from build123d import *

# Parameters (mm, degrees)
BOSS_EXTRUDE1_DEPTH     = 15.24
CUT_EXTRUDE2_DEPTH      = 2.54
CUT_EXTRUDE3_DEPTH      = 26.416
CUT_EXTRUDE4_DEPTH      = 2.54
CUT_EXTRUDE5_DEPTH      = 37.592
CUT_EXTRUDE5_DEPTH_BACK = 16.256
SKETCH6_W               = 28.095448716
SKETCH6_H               = 6.506871402
CUT_EXTRUDE6_DEPTH      = 33.782
CUT_EXTRUDE6_DEPTH_BACK = 30.988
CUT_EXTRUDE7_DEPTH      = 30.988
BOSS_EXTRUDE2_DEPTH     = 2.54


with BuildPart() as part:
    # Sketch1 → Boss-Extrude1 (new body)
    with BuildSketch(Plane(origin=(0, 0, 0), x_dir=(1, 0, 0), z_dir=(0, 1, 0))):
        Polygon((0, 0), (19.056811247, 0), (19.056811247, 6.097892911), (26.173997358, 6.097892911), (15.563225472, -28.095448716), (7.752418672, -26.383450539), (6.430712527, -32.413592092), (-14.191226065, -27.893608153), (-12.86951992, -21.8634666), (-25.576280295, -19.078357307), (-6.082744599, 6.097892911), (0, 6.097892911), align=None)
    extrude(amount=BOSS_EXTRUDE1_DEPTH)

    # Sketch2 → Cut-Extrude2 (cut)
    with BuildSketch(Plane(origin=(0, 15.24, 0), x_dir=(1, 0, 0), z_dir=(0, 1, 0))):
        Polygon((-12.86951992, -21.8634666), (7.752418672, -26.383450539), (6.430712527, -32.413592092), (-14.191226065, -27.893608153), align=None)
    extrude(amount=-CUT_EXTRUDE2_DEPTH, mode=Mode.SUBTRACT)

    # Sketch3 → Cut-Extrude3 (cut)
    with BuildSketch(Plane(origin=(12.914786435, 0, 2.830705125), x_dir=(0.214100757, 0, -0.976811582), z_dir=(0.976811582, 0, 0.214100757))):
        with BuildLine():
            Line((-29.362167954, 11.792818882), (-30.285151737, 12.7))
            Line((-30.285151737, 12.7), (-30.285151737, 6.632404251))
            Line((-30.285151737, 6.632404251), (-27.19850654, 6.632404251))
            ThreePointArc((-27.19850654, 6.632404251), (-29.99633203, 8.493128354), (-29.362167954, 11.792818882))
        make_face()
        with BuildLine():
            Line((-27.19850654, 12.7), (-30.285151737, 12.7))
            Line((-30.285151737, 12.7), (-29.362167954, 11.792818882))
            ThreePointArc((-29.362167954, 11.792818882), (-28.371580312, 12.464027615), (-27.19850654, 12.7))
        make_face()
        with BuildLine():
            ThreePointArc((-25.999973236, 9.666202125), (-26.744632367, 10.775472298), (-28.053283414, 10.506344124))
            Line((-28.053283414, 10.506344124), (-26.343729666, 8.826060127))
            ThreePointArc((-26.343729666, 8.826060127), (-26.089236367, 9.212327952), (-25.999973236, 9.666202125))
        make_face()
        with BuildLine():
            Line((-26.343729666, 8.826060127), (-28.053283414, 10.506344124))
            ThreePointArc((-28.053283414, 10.506344124), (-28.038648539, 8.811425251), (-26.343729666, 8.826060127))
        make_face()
        Polygon((-27.19850654, 6.632404251), (-30.285151737, 6.632404251), (-30.285151737, 0), (-24.111861344, 0), (-24.111861344, 6.632404251), align=None)
    extrude(amount=-CUT_EXTRUDE3_DEPTH, mode=Mode.SUBTRACT)

    # Sketch4 → Cut-Extrude4 (cut)
    with BuildSketch(Plane(origin=(0, 15.24, 0), x_dir=(1, 0, 0), z_dir=(0, 1, 0))):
        Polygon((0, 0), (0, 6.097892911), (-6.082744599, 6.097892911), (-10.804237756, 0), align=None)
        Polygon((19.056811247, 0), (24.281718113, 0), (26.173997358, 6.097892911), (19.056811247, 6.097892911), align=None)
    extrude(amount=-CUT_EXTRUDE4_DEPTH, mode=Mode.SUBTRACT)

    # Sketch5 → Cut-Extrude5 (cut, two sides)
    with BuildSketch(Plane.ZY.offset(-19.056811247)) as cut_extrude5_sk:
        with BuildLine():
            ThreePointArc((-1.900262012, 9.603435701), (-2.605255865, 10.662970793), (-3.854871247, 10.421947266))
            Line((-3.854871247, 10.421947266), (-2.243021664, 8.784924136))
            ThreePointArc((-2.243021664, 8.784924136), (-1.989411364, 9.15974511), (-1.900262012, 9.603435701))
        make_face()
        with BuildLine():
            Line((-2.243021664, 8.784924136), (-3.854871247, 10.421947266))
            ThreePointArc((-3.854871247, 10.421947266), (-3.867458021, 8.79751091), (-2.243021664, 8.784924136))
        make_face()
        with BuildLine():
            ThreePointArc((-3.048946456, 6.506871402), (-5.038116892, 7.230270846), (-6.097892911, 9.062477322))
            Line((-6.097892911, 9.062477322), (-6.097892911, 6.506871402))
            Line((-6.097892911, 6.506871402), (-3.048946456, 6.506871402))
        make_face()
        Polygon((-3.048946456, 6.506871402), (-6.097892911, 6.506871402), (-6.097892911, 0), (0, 0), (0, 6.506871402), align=None)
        with BuildLine():
            Line((-5.221516955, 11.809936977), (-6.097892911, 12.7))
            Line((-6.097892911, 12.7), (-6.097892911, 10.14439408))
            ThreePointArc((-6.097892911, 10.14439408), (-5.789305577, 11.045358842), (-5.221516955, 11.809936977))
        make_face()
        with BuildLine():
            Line((-3.048946456, 12.7), (-6.097892911, 12.7))
            Line((-6.097892911, 12.7), (-5.221516955, 11.809936977))
            ThreePointArc((-5.221516955, 11.809936977), (-4.22285816, 12.468857444), (-3.048946456, 12.7))
        make_face()
    extrude(amount=CUT_EXTRUDE5_DEPTH, mode=Mode.SUBTRACT)
    extrude(cut_extrude5_sk.sketch, amount=-CUT_EXTRUDE5_DEPTH_BACK, mode=Mode.SUBTRACT)

    # Sketch6 → Cut-Extrude6 (cut, two sides)
    with BuildSketch(Plane(origin=(0, 0, 0), x_dir=(0, 0, -1), z_dir=(1, 0, 0))) as cut_extrude6_sk:
        with Locations((-14.047724358, 3.253435701)):
            Rectangle(SKETCH6_W, SKETCH6_H)
    extrude(amount=CUT_EXTRUDE6_DEPTH, mode=Mode.SUBTRACT)
    extrude(cut_extrude6_sk.sketch, amount=-CUT_EXTRUDE6_DEPTH_BACK, mode=Mode.SUBTRACT)

    # Sketch7 → Cut-Extrude7 (cut)
    with BuildSketch(Plane(origin=(0, 15.24, 0), x_dir=(1, 0, 0), z_dir=(0, 1, 0))):
        Polygon((14.008950707, -3.834200977), (7.607295542, -3.834200977), (0.172703368, -18.672351511), (6.066325192, -20.069477121), align=None)
        Polygon((0.172703368, -18.672351511), (7.607295542, -3.834200977), (1.320524054, -3.834200977), (-6.028876319, -17.202222267), align=None)
    extrude(amount=-CUT_EXTRUDE7_DEPTH, mode=Mode.SUBTRACT)

    # Sketch8 → Boss-Extrude2 (add)
    with BuildSketch(Plane(origin=(0, 15.24, 0), x_dir=(1, 0, 0), z_dir=(0, 1, 0))):
        Polygon((-10.804237756, 0), (24.281718113, 0), (26.173997358, 6.097892911), (-6.082744599, 6.097892911), align=None)
    extrude(amount=-BOSS_EXTRUDE2_DEPTH)


solid = part.part
CAD build for the part. Positions are in the model's coordinates, mm. A direction names the side the tool comes from. Give positions to 0.01 mm unless a question says otherwise; leave off trailing zeros. Loops run counter-clockwise (first coordinate to the right, second up) from the corner with the lowest first, then second, coordinate; pieces in that order, holes last. Notation, with made-up numbers: M -15.5,-6 L 16.5,-6 A20 ccw 16.5,10 Z; hole C 63.5,35 d6. An arc over 180 degrees is marked long. Answer in a Markdown table with one row per item. Add a question column.
Item 1: Band-saw the part on B-B on y = 14. Give the cut face in (x, z), then the cut area to 3 significant figures.
Item 2: Tool access for faces 1 (the face through (-3, 12.7, 26)), 2 (the face through (-3, 6.632, 26)), 3 (the face through (9.98, 10.93, 12.07)), 4 (the face through (0, 9.6, -1.7)): list every direction of +Z, -Z, +X, -X, +Y, -Y with a clear straight run to the whole face (end or side of a thin tool).
Item 3: Mould opens along Y. For faces 5 (the face through (9, 12.7, -4)), 6 (the face through (22.6, 9.6, -6.098)), 7 (the face through (6, 15.24, 3)), 8 (the face through (-3.2, 7.2, -5)) say: +Y half, -Y half, draft (parallel to the pull), parting line (faces both ways), or undercut.
Item 4: Band-saw the part on C-C on x = 23.5. Give the cut face in (y, z).
Item 5: Probe probe 1 along Z at (x, y) = (4.5, 10.5); probe 2 along Z at (x, y) = (13, 12.5); probe 3 along Y at (x, z) = (15, -1.5). List the from-to ranges inside material, lowest first.
Item 6: Band-saw the part on A-A on z = 9.5. Give the cut face in (x, y).
Item 7: Band-saw the part on D-D on z = 23. Give the cut face in (x, y).
Item 8: Drop flat-ended pins along their axis: P1, Ø1.8, axis at x = 4.5, z = -3, coming from the -Y side; P2, Ø1, axis at y = 13, z = 12, coming from the -X side; P3, Ø1, axis at x = -11, y = 11.5, coming from the -Z side. Give the stop position or say it passes through.
Reply:
| question | item | result |
|---|---|---|
| 1 | outline | M -25.58,19.08 L -6.08,-6.1 L 26.17,-6.1 L 15.56,28.1 Z; hole M -6.03,17.2 L 1.32,3.83 L 14.01,3.83 L 6.07,20.07 Z |
| 1 | area | 963 mm^2 |
| 2 | face 1 | +Z, -X, +Y |
| 2 | face 2 | +Z, -X, -Y |
| 2 | face 3 | +Y, -Y |
| 2 | face 4 | -Z, -Y |
| 3 | face 5 | undercut |
| 3 | face 6 | draft |
| 3 | face 7 | +Y half |
| 3 | face 8 | -Y half |
| 4 | outline | M 6.51,-3.05 A3.1 ccw 9.06,-6.1 L 10.14,-6.1 A3.1 ccw 12.7,-3.05 L 12.7,-6.1 L 15.24,-6.1 L 15.24,2.52 L 6.51,2.52 Z; hole C 9.6,-3.05 d2.3 |
| 5 | probe 1 | z = 0 to 3.83, 19.7 to 27.95, 29.71 to 31.82 |
| 5 | probe 2 | z = 0 to 3.83, 5.9 to 27.53 |
| 5 | probe 3 | y = 12.7 to 15.24 |
| 6 | outline | M -18.16,6.51 L -1.79,6.51 L -1.79,15.24 L -18.16,15.24 Z; M 11.24,6.51 L 21.33,6.51 L 21.33,15.24 L 11.24,15.24 Z |
| 7 | outline | M -13.12,6.63 L -7.68,6.63 L -7.68,6.51 L 17.14,6.51 L 17.14,15.24 L -7.68,15.24 L -7.68,12.7 L -13.12,12.7 Z |
| 8 | P1 | stops at y = 12.7 |
| 8 | P2 | stops at x = -20.48 |
| 8 | P3 | stops at z = -0.39 |
